```python
from build123d import *

# Parameters (mm, degrees)
SKETCH2_R          = 2
CUT_EXTRUDE1_DEPTH = 10


with BuildPart() as part:
    # Sketch1 → Revolve1 (revolve)
    with BuildSketch(Plane.XY):
        Polygon((0, 0), (0, 16), (-5.5, 16), (-5.5, 14.5), (-3.61, 14.5), (-3.61, 7.1), (-5.5, 7.1), (-5.5, 0), align=None)
    revolve(axis=Axis((2.5, 19.494779208, 0), (0, -1, 0)))

    # Sketch2 → Cut-Extrude1 (cut)
    with BuildSketch(Plane.XY):
        with Locations((2.5, 3.55)):
            Circle(SKETCH2_R)
    extrude(amount=CUT_EXTRUDE1_DEPTH, mode=Mode.SUBTRACT)


solid = part.part
```
Source: CAD feature listing. Evaluate the final solid. Frame: model axes, mm. A direction names the side the tool comes from. Give positions to 0.01 mm unless a question says otherwise; leave off trailing zeros. Loops run counter-clockwise (first coordinate to the right, second up) from the corner with the lowest first, then second, coordinate; pieces in that order, holes last. Notation, with made-up numbers: (-24.5, 87) -> (32.5, 87) arc R14 ccw to (32.5, 112) -> close; hole circle Ø2 at (56.25, 74). An arc over 180 degrees is marked (long way). Put each result on its own line as item: value. Start each with the question number.
1) Cut plane C-C (z = 5). Return loops of the section in (x, y) (3 decimals).
2) Cut plane A-A (x = 2.5). Return loops of the section in (y, z).
3) Material intervals for probe 1 along Y at (x, z) = (2.5, 6.75); probe 2 along Z at (x, y) = (2.5, 9.5); probe 3 along Y at (x, z) = (2.5, 4.75), sorted ascending.
4) Cut plane D-D (x = 6). Return loops of the section in (y, z), then the cut area to 3 significant figures.
5) Draft query along Z for faces 1 (the face through (8, 14.5, 3)), 2 (the face through (2.83, 8.11, -2.48)), 3 (the face through (-1.801, 3.5, -6.746)). Return one class per face: released by +Z, released by -Z, zero draft, split by the parting line, or undercut.
6) Cut plane B-B (z = 0). Return loops of the section in (x, y), then the cut area to 3 significant figures.
7) Reachability of faces 4 (the face through (-3, 7.1, 3)), 5 (the face through (4.23, 15.24, 7.81)), 6 (the face through (4.408, 4.151, 4.708)) from +Z, -Z, +X, -X, +Y, -Y: full face, straight path, thin tool, end or side. Return the list, or none.
8) Contact query for flat-ended pins moving along their axis: P1, Ø1, axis at y = 3.5, z = 1, coming from the +X side; P2, Ø1.5, axis at x = 5.5, y = 3, coming from the +Z side; P3, Ø3, axis at x = -0.5, y = 3.5, coming from the -Z side. Output: stop coordinate, or through.
Results are:
1. outline: (-3.745, 0) -> (8.745, 0) -> (8.745, 7.1) -> (6.012, 7.1) -> (6.012, 14.5) -> (8.745, 14.5) -> (8.745, 16) -> (-3.745, 16) -> (-3.745, 14.5) -> (-1.012, 14.5) -> (-1.012, 7.1) -> (-3.745, 7.1) -> close; hole circle Ø4 at (2.5, 3.55)
2. outline: (0, -8) -> (7.1, -8) -> (7.1, -6.11) -> (14.5, -6.11) -> (14.5, -8) -> (16, -8) -> (16, -2.5) -> (0, -2.5) -> close; (0, 2.5) -> (1.55, 2.5) -> (1.55, 8) -> (0, 8) -> close; (5.55, 2.5) -> (16, 2.5) -> (16, 8) -> (14.5, 8) -> (14.5, 6.11) -> (7.1, 6.11) -> (7.1, 8) -> (5.55, 8) -> close
3. probe 1: y = 0 to 1.55, 5.55 to 7.1, 14.5 to 16
3. probe 2: z = -6.11 to -2.5, 2.5 to 6.11
3. probe 3: y = 0 to 1.55, 5.55 to 16
4. outline: (0, -7.19) -> (7.1, -7.19) -> (7.1, -5.01) -> (14.5, -5.01) -> (14.5, -7.19) -> (16, -7.19) -> (16, 7.19) -> (14.5, 7.19) -> (14.5, 5.01) -> (7.1, 5.01) -> (7.1, 7.19) -> (0, 7.19) -> close
4. area: 198 mm2
5. face 1: zero draft
5. face 2: undercut
5. face 3: split by the parting line
6. outline: (-5.5, 0) -> (0, 0) -> (0, 16) -> (-5.5, 16) -> (-5.5, 14.5) -> (-3.61, 14.5) -> (-3.61, 7.1) -> (-5.5, 7.1) -> close; (5, 0) -> (10.5, 0) -> (10.5, 7.1) -> (8.61, 7.1) -> (8.61, 14.5) -> (10.5, 14.5) -> (10.5, 16) -> (5, 16) -> close
6. area: 148 mm2
7. face 4: none
7. face 5: +Y, -Y
7. face 6: +Z
8. P1: stops at x = 10.48
8. P2: stops at z = 7.68
8. P3: stops at z = -7.86
